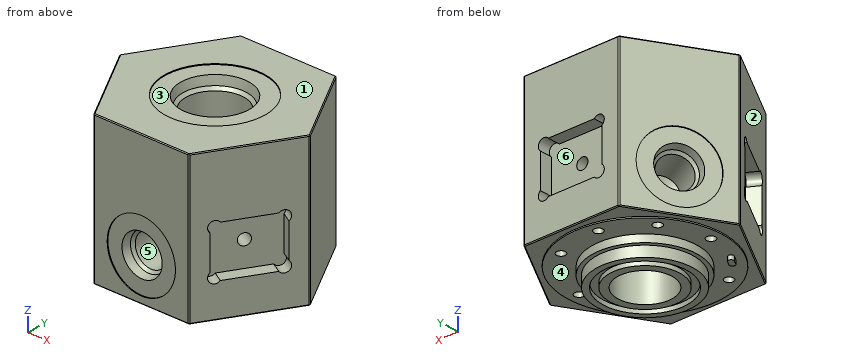
from build123d import *

# Parameters (mm, degrees)
SKETCH1_R                 = 8.255
BOSS_EXTRUDE1_DEPTH       = 44.45
CHAMFER1_SIZE             = 0.254
CHAMFER2_SIZE             = 0.254
CUT_EXTRUDE16_DEPTH       = 3.81
CIRPATTERN3_COUNT         = 3
CIRPATTERN4_COUNT         = 2
CIRPATTERN4_ANGLE         = 120
CIRPATTERN5_COUNT         = 3
CIRPATTERN6_COUNT         = 2
CIRPATTERN6_ANGLE         = 60
CIRPATTERN7_COUNT         = 2
F_6_32_TAPPED_HOLE2_D     = 2.7051
F_6_32_TAPPED_HOLE2_DEPTH = 6.35
F_6_32_TAPPED_HOLE2_TIP   = 0.81269403
BOSS_EXTRUDE2_DEPTH       = 1.27
CHAMFER3_SIZE             = 0.254
CHAMFER3_EDGE_2_SIZE      = 0.254
CHAMFER3_EDGE_3_SIZE      = 0.254
CHAMFER3_EDGE_4_SIZE      = 0.254
CHAMFER3_EDGE_5_SIZE      = 0.254
CHAMFER3_EDGE_6_SIZE      = 0.254
SKETCH60_R                = 1.74625
CUT_EXTRUDE17_DEPTH       = 3.81
MIRROR2_COPY_1_SKETCH_R   = 1.74625
MIRROR2_COPY_1_DEPTH      = 3.81
SKETCH61_R                = 1.74625
CUT_EXTRUDE18_DEPTH       = 3.81
MIRROR4_COPY_1_SKETCH_R   = 1.74625
MIRROR4_COPY_1_DEPTH      = 3.81
SKETCH62_R                = 1.74625
CUT_EXTRUDE19_DEPTH       = 3.81
MIRROR6_COPY_1_SKETCH_R   = 1.74625
MIRROR6_COPY_1_DEPTH      = 3.81


with BuildPart() as part:
    # Sketch1 → Boss-Extrude1 (new body)
    with BuildSketch(Plane.XY):
        Polygon((29.329393675, 0), (14.664696837, 25.4), (-14.664696837, 25.4), (-29.329393675, 0), (-14.664696837, -25.4), (14.664696837, -25.4), align=None)
        Circle(SKETCH1_R, mode=Mode.SUBTRACT)
    extrude(amount=BOSS_EXTRUDE1_DEPTH)

    # Chamfer1
    chamfer1_edges = [part.edges().sort_by_distance(p)[0] for p in [
        (0, 25.4, 44.45),
        (-21.997045256, 12.7, 44.45),
        (-21.997045256, -12.7, 44.45),
        (0, -25.4, 44.45),
        (21.997045256, -12.7, 44.45),
        (21.997045256, 12.7, 44.45),
    ]]
    chamfer(chamfer1_edges, length=CHAMFER1_SIZE)

    # Chamfer2
    chamfer2_edges = [part.edges().sort_by_distance(p)[0] for p in [
        (0, -25.4, 0),
        (-21.997045256, -12.7, 0),
        (-21.997045256, 12.7, 0),
        (0, 25.4, 0),
        (21.997045256, 12.7, 0),
        (21.997045256, -12.7, 0),
    ]]
    chamfer(chamfer2_edges, length=CHAMFER2_SIZE)

    # Sketch42 → Cut-Extrude16 (cut)
    with BuildSketch(Plane(origin=(0, 25.4, 0), x_dir=(1, 0, 0), z_dir=(0, 1, 0))):
        with BuildLine():
            Line((-7.62, -10.2108), (7.62, -10.2108))
            ThreePointArc((7.62, -10.2108), (8.967038418, -10.768761582), (9.525, -12.1158))
            Line((9.525, -12.1158), (9.525, -23.5458))
            ThreePointArc((9.525, -23.5458), (8.967038418, -24.892838418), (7.62, -25.4508))
            Line((7.62, -25.4508), (-7.62, -25.4508))
            ThreePointArc((-7.62, -25.4508), (-8.967038418, -24.892838418), (-9.525, -23.5458))
            Line((-9.525, -23.5458), (-9.525, -12.1158))
            ThreePointArc((-9.525, -12.1158), (-8.967038418, -10.768761582), (-7.62, -10.2108))
        make_face()
    cut_extrude16 = extrude(amount=-CUT_EXTRUDE16_DEPTH, mode=Mode.SUBTRACT)

    # Sketch43 → Cut-Revolve1 (revolve, cut)
    with BuildSketch(Plane(origin=(0, 0, 0), x_dir=(1, 0, 0), z_dir=(0, 1, 0)), mode=Mode.PRIVATE) as cut_revolve1_sk:
        Polygon((10.2997, -44.196), (9.619109051, -41.656), (8.7376, -40.774490949), (8.7376, -23.299290949), (4.9657, -21.121583468), (0, -21.121583468), (0, -44.45), (15.0876, -44.45), (15.0876, -44.196), align=None)
    revolve(cut_revolve1_sk.sketch.rotate(Axis((0, 0, 44.45), (0, 0, 1)), 180), axis=Axis((0, 0, 44.45), (0, 0, 1)), mode=Mode.SUBTRACT)

    # CirPattern3: Cut-Extrude16 ×3 about axis
    cirpattern3_axis = Axis((0, 0, 0), (0, 0, 1))
    for i in range(1, CIRPATTERN3_COUNT):
        add(cut_extrude16.rotate(cirpattern3_axis, i * 360 / CIRPATTERN3_COUNT), mode=Mode.SUBTRACT)

    # Sketch44 → Cut-Revolve2 (revolve, cut)
    with BuildSketch(Plane.XY.offset(12.7), mode=Mode.PRIVATE) as cut_revolve2_sk:
        Polygon((-24.856484742, 7.209190797), (-22.559708978, 6.462923113), (-21.493391064, 6.748642137), (-12.182750987, 1.373141582), (-9.464950987, 2.942264144), (-2.86583741, -0.867735856), (-1.77363741, 1.024010036), (-21.764034742, 12.565471317), (-21.997045256, 12.7), (-27.254845256, 3.593223264), (-27.021834742, 3.458694581), align=None)
    cut_revolve2 = revolve(cut_revolve2_sk.sketch.rotate(Axis((-1.77363741, 1.024010036, 12.7), (-0.8660254037844387, 0.5, 0)), 180), axis=Axis((-1.77363741, 1.024010036, 12.7), (-0.8660254037844387, 0.5, 0)), mode=Mode.SUBTRACT)

    # CirPattern4: Cut-Revolve2 ×2 about axis
    cirpattern4_axis = Axis((0, 0, 0), (0, 0, 1))
    for i in range(1, CIRPATTERN4_COUNT):
        add(cut_revolve2.rotate(cirpattern4_axis, i * CIRPATTERN4_ANGLE / (CIRPATTERN4_COUNT - 1)), mode=Mode.SUBTRACT)

    # Sketch47 → #8-32 Tapped Hole1 (revolve, cut)
    with BuildSketch(Plane(origin=(-18.697488468, -10.795, 17.8308), x_dir=(0.5000000000000042, -0.8660254037844362, 0), z_dir=(0, 0, 1))):
        Polygon((0, 0), (0, 11.197806461), (1.7272, 10.16), (1.7272, 0), align=None)
    f_8_32_tapped_hole1 = revolve(axis=Axis((-24.196749782, -13.97, 17.8308), (0.8660254037844362, 0.5000000000000042, 0)), mode=Mode.SUBTRACT)

    # CirPattern5: #8-32 Tapped Hole1 ×3 about axis
    cirpattern5_axis = Axis((0, 0, 0), (0, 0, 1))
    for i in range(1, CIRPATTERN5_COUNT):
        add(f_8_32_tapped_hole1.rotate(cirpattern5_axis, i * 360 / CIRPATTERN5_COUNT), mode=Mode.SUBTRACT)

    # Sketch49 → Revolve1 (revolve)
    with BuildSketch(Plane(origin=(0, 0, 0), x_dir=(0, 0, -1), z_dir=(1, 0, 0)), mode=Mode.PRIVATE) as revolve1_sk:
        Polygon((0, 23.622), (0, 8.255), (5.842, 8.255), (5.842, 10.6172), (4.5466, 10.6172), (4.5466, 12.7508), (5.842, 12.7508), (5.842, 14.605), (2.667, 14.605), (2.667, 15.84325), (0.381, 15.84325), (0.381, 23.622), align=None)
    revolve(revolve1_sk.sketch.rotate(Axis((0, 0, 0), (0, 0, -1)), 90), axis=Axis((0, 0, 0), (0, 0, -1)))

    # Sketch25 → #6-32 Tapped Hole1 (revolve, cut)
    with BuildSketch(Plane(origin=(-20.32, 0, -0.381), x_dir=(0, 1, 0), z_dir=(1, 0, 0))):
        Polygon((0, 0), (0, 7.16269403), (1.35255, 6.35), (1.35255, 0), align=None)
    f_6_32_tapped_hole1 = revolve(axis=Axis((-20.32, 0, -6.731), (0, 0, 1)), mode=Mode.SUBTRACT)

    # CirPattern6: #6-32 Tapped Hole1 ×2 about axis
    cirpattern6_axis = Axis((0, 0, -5.842), (0, 0, 1))
    for i in range(1, CIRPATTERN6_COUNT):
        add(f_6_32_tapped_hole1.rotate(cirpattern6_axis, i * CIRPATTERN6_ANGLE / (CIRPATTERN6_COUNT - 1)), mode=Mode.SUBTRACT)

    # CirPattern7: #6-32 Tapped Hole1 ×2 about axis
    cirpattern7_axis = Axis((0, 0, 0), (0, 0, 1))
    for i in range(1, CIRPATTERN7_COUNT):
        add(f_6_32_tapped_hole1.rotate(cirpattern7_axis, i * 360 / CIRPATTERN7_COUNT), mode=Mode.SUBTRACT)

    # CirPattern7 copy 1 sketch → CirPattern7 copy 1 (revolve, cut)
    with BuildSketch(Plane(origin=(10.16, 17.597636205, -0.381), x_dir=(0.8660254037844397, -0.4999999999999981, 0), z_dir=(-0.4999999999999981, -0.8660254037844397, 0))):
        Polygon((0, 0), (0, 7.16269403), (1.35255, 6.35), (1.35255, 0), align=None)
    revolve(axis=Axis((10.16, 17.597636205, -6.731), (0, 0, 1)), mode=Mode.SUBTRACT)

    # #6-32 Tapped Hole2
    with Locations(Plane(origin=(0, 0, -0.381), x_dir=(-1, 0, 0), z_dir=(0, 0, -1))):
        with Locations((15.566023084, 13.061444229), (3.52853097, 20.011293541), (-15.566023084, -13.061444229), (-3.52853097, -20.011293541)):
            Hole(F_6_32_TAPPED_HOLE2_D / 2, depth=F_6_32_TAPPED_HOLE2_DEPTH)
            with Locations((0, 0, -(F_6_32_TAPPED_HOLE2_DEPTH + F_6_32_TAPPED_HOLE2_TIP / 2))):  # 118° drill point
                Cone(0, F_6_32_TAPPED_HOLE2_D / 2, F_6_32_TAPPED_HOLE2_TIP, mode=Mode.SUBTRACT)

    # Sketch50 → Boss-Extrude2 (add)
    with BuildSketch(Plane(origin=(0, 0, -0.381), x_dir=(-1, 0, 0), z_dir=(0, 0, -1))):
        with BuildLine():
            Line((16.508829575, -10.440588403), (17.296229575, -9.076771597))
            ThreePointArc((17.296229575, -9.076771597), (18.392656205, -8.782984967), (18.686442835, -9.879411597))
            Line((18.686442835, -9.879411597), (17.899042835, -11.243228403))
            ThreePointArc((17.899042835, -11.243228403), (16.802616205, -11.537015033), (16.508829575, -10.440588403))
        make_face()
    extrude(amount=BOSS_EXTRUDE2_DEPTH)

    # Chamfer3
    chamfer3_edges = [part.edges().sort_by_distance(p)[0] for p in [
        (14.664696837, -25.4, 22.225),
    ]]
    chamfer(chamfer3_edges, length=CHAMFER3_SIZE)

    # Chamfer3 edge 2
    chamfer3_edge_2_edges = [part.edges().sort_by_distance(p)[0] for p in [
        (-14.664696837, -25.4, 22.225),
    ]]
    chamfer(chamfer3_edge_2_edges, length=CHAMFER3_EDGE_2_SIZE)

    # Chamfer3 edge 3
    chamfer3_edge_3_edges = [part.edges().sort_by_distance(p)[0] for p in [
        (-29.329393675, 0, 22.225),
    ]]
    chamfer(chamfer3_edge_3_edges, length=CHAMFER3_EDGE_3_SIZE)

    # Chamfer3 edge 4
    chamfer3_edge_4_edges = [part.edges().sort_by_distance(p)[0] for p in [
        (-14.664696837, 25.4, 22.225),
    ]]
    chamfer(chamfer3_edge_4_edges, length=CHAMFER3_EDGE_4_SIZE)

    # Chamfer3 edge 5
    chamfer3_edge_5_edges = [part.edges().sort_by_distance(p)[0] for p in [
        (14.664696837, 25.4, 22.225),
    ]]
    chamfer(chamfer3_edge_5_edges, length=CHAMFER3_EDGE_5_SIZE)

    # Chamfer3 edge 6
    chamfer3_edge_6_edges = [part.edges().sort_by_distance(p)[0] for p in [
        (29.329393675, 0, 22.225),
    ]]
    chamfer(chamfer3_edge_6_edges, length=CHAMFER3_EDGE_6_SIZE)

    # Sketch60 → Cut-Extrude17 (cut)
    with BuildSketch(Plane(origin=(0, 25.4, 0), x_dir=(1, 0, 0), z_dir=(0, 1, 0))):
        with Locations((-8.413693305, -11.322106695)):
            Circle(SKETCH60_R)
    cut_extrude17 = extrude(amount=-CUT_EXTRUDE17_DEPTH, mode=Mode.SUBTRACT)

    # Mirror1: Cut-Extrude17 across plane
    add(cut_extrude17.mirror(Plane(origin=(0, 0, 0), x_dir=(0, 0, 1), z_dir=(1, 0, 0))), mode=Mode.SUBTRACT)

    # Mirror2: Cut-Extrude17 across plane
    add(cut_extrude17.mirror(Plane.XY.offset(17.8308)), mode=Mode.SUBTRACT)

    # Mirror2 copy 1 sketch → Mirror2 copy 1 (cut)
    with BuildSketch(Plane(origin=(0, 25.4, 35.6616), x_dir=(-1, 0, 0), z_dir=(0, 1, 0))):
        with Locations((-8.413693305, -11.322106695)):
            Circle(MIRROR2_COPY_1_SKETCH_R)
    extrude(amount=-MIRROR2_COPY_1_DEPTH, mode=Mode.SUBTRACT)

    # Sketch61 → Cut-Extrude18 (cut)
    with BuildSketch(Plane(origin=(-21.997045256, -12.7, 0), x_dir=(0, 0, 1), z_dir=(-0.8660254037844388, -0.49999999999999967, 0))):
        with Locations((24.339493305, 8.413693305)):
            Circle(SKETCH61_R)
    cut_extrude18 = extrude(amount=-CUT_EXTRUDE18_DEPTH, mode=Mode.SUBTRACT)

    # Mirror3: Cut-Extrude18 across plane
    add(cut_extrude18.mirror(Plane(origin=(0, 0, 0), x_dir=(0, 0, 1), z_dir=(0.5000000000000041, -0.8660254037844364, 0))), mode=Mode.SUBTRACT)

    # Mirror4: Cut-Extrude18 across plane
    add(cut_extrude18.mirror(Plane(origin=(0, 0, 17.8308), x_dir=(1, 0, 0), z_dir=(0, 0, -1))), mode=Mode.SUBTRACT)

    # Mirror4 copy 1 sketch → Mirror4 copy 1 (cut)
    with BuildSketch(Plane(origin=(-21.997045256, -12.7, 35.6616), x_dir=(0, 0, -1), z_dir=(-0.8660254037844337, -0.5000000000000084, 0))):
        with Locations((24.339493305, 8.413693305)):
            Circle(MIRROR4_COPY_1_SKETCH_R)
    extrude(amount=-MIRROR4_COPY_1_DEPTH, mode=Mode.SUBTRACT)

    # Sketch62 → Cut-Extrude19 (cut)
    with BuildSketch(Plane(origin=(21.997045256, -12.7, 0), x_dir=(0, 0, -1), z_dir=(0.8660254037844389, -0.49999999999999983, 0))):
        with Locations((-24.339493305, -8.413693305)):
            Circle(SKETCH62_R)
    cut_extrude19 = extrude(amount=-CUT_EXTRUDE19_DEPTH, mode=Mode.SUBTRACT)

    # Mirror5: Cut-Extrude19 across plane
    add(cut_extrude19.mirror(Plane(origin=(0, 0, 0), x_dir=(0, 0, 1), z_dir=(0.49999999999999195, 0.8660254037844434, 0))), mode=Mode.SUBTRACT)

    # Mirror6: Cut-Extrude19 across plane
    add(cut_extrude19.mirror(Plane(origin=(0, 0, 17.8308), x_dir=(1, 0, 0), z_dir=(0, 0, -1))), mode=Mode.SUBTRACT)

    # Mirror6 copy 1 sketch → Mirror6 copy 1 (cut)
    with BuildSketch(Plane(origin=(21.997045256, -12.7, 35.6616), x_dir=(0, 0, 1), z_dir=(0.8660254037844479, -0.4999999999999841, 0))):
        with Locations((-24.339493305, -8.413693305)):
            Circle(MIRROR6_COPY_1_SKETCH_R)
    extrude(amount=-MIRROR6_COPY_1_DEPTH, mode=Mode.SUBTRACT)


solid = part.part
Verification items for the finished model (mm, model axes). Face numbers are marked on the shaded views. A direction names the side the tool comes from. Round coordinates to 2 decimals unless told otherwise and drop trailing zeros.
(1) Mould release check, pull along Y, two halves, no side actions. Record for the marked faces 1, 2 and 3: pulls with the +Y half, pulls with the -Y half, needs draft (parallel to the pull), parting line crosses it, or undercut.
Returned:
face 1: needs draft
face 2: pulls with the -Y half
face 3: undercut
(2) Depth check by flat-ended pin: pin 1 Ø6 at (y, z) = (11.5, 26) entering from +X; pin 2 Ø10 at (y, z) = (-17.5, 34.5) entering from -X; pin 3 Ø9 at (x, y) = (-6.5, -2) entering from +Z; pin 4 Ø10.5 at (x, y) = (0, 0) entering from +Z. Enter the tip coordinate at first touch or a pass-through.
Returned:
pin 1: stops at x = 24.42
pin 2: stops at x = -22.11
pin 3: stops at z = 44.2
pin 4: passes through
(3) Access from +Z, -Z, +X, -X, +Y, -Y to the whole of each face (thin tool, end or side, straight path). Record for the marked faces 4, 5 and 6.
Returned:
face 4: -Z
face 5: -Y
face 6: +Y
(4) Material ranges on line 1 (Y direction, x = 0, z = -5) (3 decimals); line 2 (Z direction, x = 0, y = -16.5); line 3 (Y direction, x = -10, z = 2), recorded low to high.
Returned:
line 1: y = -14.605 to -12.751, -10.617 to -8.255, 8.255 to 10.617, 12.751 to 14.605
line 2: z = -0.38 to 7.8, 17.6 to 44.45
line 3: y = -25.4 to -18.94, -16.25 to 25.4
